Input: part model. Units: mm. Frame: model coordinates. A direction names the side the tool comes from. Give positions to 0.01 mm unless a question says otherwise; leave off trailing zeros. Order: outer loops, then holes, each group sorted by start corner. A loop starts at its lowest first (then second) coordinate and runs counter-clockwise, first axis right, second up. Notation, with made-up numbers: (65, 52.25) - (106, 52.25) arc R34 ccw to (106, 87.25) - close; hole circle Ø5 at (-3.5, -15). An arc over 180 degrees is marked (long way). Answer in a Markdown table with one row per item. Add a question column.
1. Ray query, line 1 (Z direction, x = 0, y = 0.45); line 2 (X direction, y = 6, z = 0). Return the intervals inside material, ascending. Write a range as [from, to].
2. Contact query for flat-ended pins moving along their axis: pin 1 (3 mm diameter, centred on x = -1, y = 1.5, fed in from +Z); pin 2 (3 mm diameter, centred on x = 3.5, y = 4.5, fed in from -Z); pin 3 (4 mm diameter, centred on y = 4, z = -3, fed in from +X). Output: stop coordinate, or through.
3. Section query C-C on x = 0. Return loops of the section in (y, z), and give its area (3 significant figures).
4. Section query B-B on y = 6. Return loops of the section in (x, z).
5. Mould query, pull axis X, two halves, no side actions, for faces 4 (the face through (0, 5, 0)), 5 (the face through (3, 7, 0)), 6 (the face through (-6, 3, 0)). Classes: released by +X, released by -X, zero draft, split by the parting line, or undercut.
6. Section query D-D on y = 2.25. Return loops of the section in (x, z), and give its area (3 significant figures).
7. Section query A-A on z = 0. Return loops of the section in (x, y).
8. Access query for faces 1 (the face through (-0.217, 0.493, -0.976)), 2 (the face through (1.2, 0, -0.1)), 3 (the face through (-0.54, 6.01, 2.44)). Directions: +Z, -Z, +X, -X, +Y, -Y. A direction counts if a zero-diameter tool reaches every point of the face in a straight line with its end or side. Return the directions, or none.
```python
from build123d import *

# Parameters (mm, degrees)
SKETCH1_R           = 6
BOSS_EXTRUDE1_DEPTH = 7
SKETCH2_R           = 2.5
CUT_EXTRUDE1_DEPTH  = 2
SKETCH4_R           = 1
CUT_EXTRUDE3_DEPTH  = 2
FILLET1_R           = 1


with BuildPart() as part:
    # Sketch1 → Boss-Extrude1 (new body)
    with BuildSketch(Plane(origin=(0, 0, 0), x_dir=(1, 0, 0), z_dir=(0, 1, 0))):
        Circle(SKETCH1_R)
    extrude(amount=BOSS_EXTRUDE1_DEPTH)

    # Sketch2 → Cut-Extrude1 (cut)
    with BuildSketch(Plane(origin=(0, 7, 0), x_dir=(1, 0, 0), z_dir=(0, 1, 0))):
        Circle(SKETCH2_R)
    extrude(amount=-CUT_EXTRUDE1_DEPTH, mode=Mode.SUBTRACT)

    # Sketch4 → Cut-Extrude3 (cut)
    with BuildSketch(Plane.XZ):
        Circle(SKETCH4_R)
    extrude(amount=-CUT_EXTRUDE3_DEPTH, mode=Mode.SUBTRACT)

    # Fillet1
    fillet1_edges = [part.edges().sort_by_distance(p)[0] for p in [
        (-1, 2, 0),
    ]]
    fillet(fillet1_edges, radius=FILLET1_R)


solid = part.part
```
Answer:
| question | item | result |
|---|---|---|
| 1 | line 1 | z = [-6, -1], [1, 6] |
| 1 | line 2 | x = [-6, -2.5], [2.5, 6] |
| 2 | pin 1 | stops at z = 6 |
| 2 | pin 2 | stops at z = -5.66 |
| 2 | pin 3 | stops at x = 5.92 |
| 3 | outline | (0, -6) - (7, -6) - (7, -2.5) - (5, -2.5) - (5, 2.5) - (7, 2.5) - (7, 6) - (0, 6) - (0, 1) - (1, 1) arc R1 cw to (1, -1) - (0, -1) - close |
| 3 | area | 70.4 mm² |
| 4 | outline | circle Ø12 at (0, 0); hole circle Ø5 at (0, 0) |
| 5 | face 4 | undercut |
| 5 | face 5 | zero draft |
| 5 | face 6 | split by the parting line |
| 6 | outline | circle Ø12 at (0, 0) |
| 6 | area | 113 mm² |
| 7 | outline | (-6, 0) - (-1, 0) - (-1, 1) arc R1 cw to (1, 1) - (1, 0) - (6, 0) - (6, 7) - (2.5, 7) - (2.5, 5) - (-2.5, 5) - (-2.5, 7) - (-6, 7) - close |
| 8 | face 1 | -Y |
| 8 | face 2 | +Z, -Z, +X, -X, -Y |
| 8 | face 3 | +Y |
